Part model, mm, in its own coordinate system. Face numbers are marked on the shaded views. A direction names the side the tool comes from. Round coordinates to 2 decimals unless told otherwise and drop trailing zeros. Write each loop counter-clockwise with the first axis right and the second up, starting at its lowest first coordinate (ties: lowest second). Pieces come first, ordered by that corner, then holes. Notation, with made-up numbers: M 74,60 L 96,60 A26 ccw 96,93 Z; hole C 32,0.25 d9. An arc over 180 degrees is marked long. Use one line per item in the form item = value. Start each with the question number.
Item 1: Cut at C-C, the plane z = 11. Give the cut face in (x, y), then the cut area to 3 significant figures.
Item 2: Which spindle directions (+Z, -Z, +X, -X, +Y, -Y) get a long thin tool onto all of the face, cutting with end or side? Do the marked faces 5 and 6. Say none if no direction does.
Item 3: Flat gauge pins, fed straight in: pin 1 Ø4 at (x, y) = (10.5, -2.5) entering from +Z; pin 2 Ø4 at (x, y) = (-7.5, 8) entering from +Z. Where does each tip first touch, or does it go through?
Item 4: Cut at B-B, the plane y = 0. Give the cut face in (x, z), then the cut area to 3 significant figures.
Item 5: Mould opens along X. For the marked faces 1, 2, 3 and 4 say: +X half, -X half, draft (parallel to the pull), parting line (faces both ways), or undercut.
Item 6: Cut at A-A, the plane z = 2.25. Give the cut face in (x, y).
Item 7: Probe L1, parallel to Y at x = -14, z = 17; L2, parallel to X at y = 0.25, z = 3; L3, parallel to Z at x = 23.1, y = 0. List the from-to ranges inside material, lowest first.
Item 8: Cut at D-D, the plane x = 8. Give the cut face in (y, z), then the cut area to 3 significant figures.
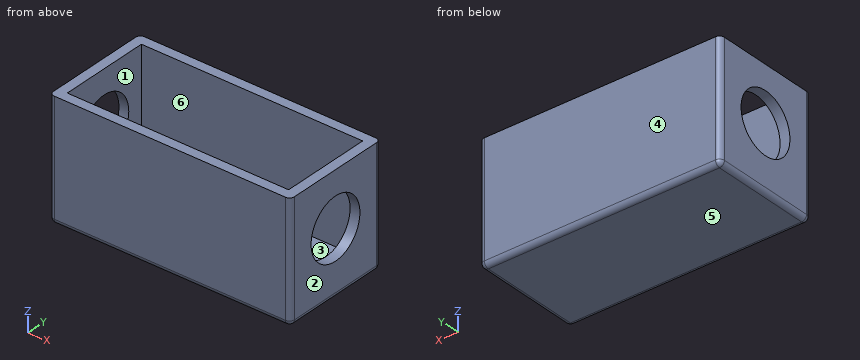
from build123d import *

# Parameters (mm, degrees)
F0_W     = 49
F0_H     = 22.5
F0_W_2   = 45
F0_H_2   = 18.5
F1_DEPTH = 22
F2_W     = 49
F2_H     = 22.5
F3_DEPTH = 2
F4_R     = 6.1
F5_DEPTH = 49.001
F6_R     = 1


with BuildPart() as f1:
    # F0 (on Top) → F1 (new body)
    with BuildSketch(Plane.XY):
        Rectangle(F0_W, F0_H)
        Rectangle(F0_W_2, F0_H_2, mode=Mode.SUBTRACT)
    extrude(amount=F1_DEPTH)

    # F2 (on face) → F3 (join)
    with BuildSketch(Plane(origin=(0, 0, 0), x_dir=(1, 0, 0), z_dir=(0, 0, -1))):
        Rectangle(F2_W, F2_H)
    extrude(amount=F3_DEPTH)

    # F4 (on face) → F5 (cut, through all)
    with BuildSketch(Plane.YZ.offset(24.5)):
        with Locations((0, 11)):
            Circle(F4_R)
    extrude(amount=-F5_DEPTH, mode=Mode.SUBTRACT)

    # F6
    f6_edges = [f1.edges().sort_by_distance(p)[0] for p in [
        (24.5, -11.25, 10),
        (24.5, 11.25, 10),
        (24.5, 0, -2),
        (0, 11.25, -2),
        (0, -11.25, -2),
        (-24.5, -11.25, 10),
        (-24.5, 0, -2),
        (-24.5, 11.25, 10),
    ]]
    fillet(f6_edges, radius=F6_R)


solid = f1.part
Model answer:
q1.outline = M -24.5,-10.25 A1 ccw -23.5,-11.25 L 23.5,-11.25 A1 ccw 24.5,-10.25 L 24.5,-6.1 L 22.5,-6.1 L 22.5,-9.25 L -22.5,-9.25 L -22.5,-6.1 L -24.5,-6.1 Z; M -24.5,6.1 L -22.5,6.1 L -22.5,9.25 L 22.5,9.25 L 22.5,6.1 L 24.5,6.1 L 24.5,10.25 A1 ccw 23.5,11.25 L -23.5,11.25 A1 ccw -24.5,10.25 Z
q1.area = 220 mm²
q2.face_5 = -Z, +X, -X, +Y, -Y
q2.face_6 = +Z
q3.pin_1 = 0
q3.pin_2 = 22
q4.outline = M -24.5,-1 A1 ccw -23.5,-2 L 23.5,-2 A1 ccw 24.5,-1 L 24.5,4.9 L 22.5,4.9 L 22.5,0 L -22.5,0 L -22.5,4.9 L -24.5,4.9 Z; M -24.5,17.1 L -22.5,17.1 L -22.5,22 L -24.5,22 Z; M 22.5,17.1 L 24.5,17.1 L 24.5,22 L 22.5,22 Z
q4.area = 137 mm²
q5.face_1 = undercut
q5.face_2 = +X half
q5.face_3 = undercut
q5.face_4 = draft
q6.outline = M -24.5,-10.25 A1 ccw -23.5,-11.25 L 23.5,-11.25 A1 ccw 24.5,-10.25 L 24.5,10.25 A1 ccw 23.5,11.25 L -23.5,11.25 A1 ccw -24.5,10.25 Z; hole M -22.5,-9.25 L 22.5,-9.25 L 22.5,9.25 L -22.5,9.25 Z
q7.L1 = -11.25 to -9.25, 9.25 to 11.25
q7.L2 = -24.5 to -22.5, 22.5 to 24.5
q7.L3 = -2 to 4.9, 17.1 to 22
q8.outline = M -11.25,-1 A1 ccw -10.25,-2 L 10.25,-2 A1 ccw 11.25,-1 L 11.25,22 L 9.25,22 L 9.25,0 L -9.25,0 L -9.25,22 L -11.25,22 Z
q8.area = 133 mm²
